Read the model definition and answer for the solid it produces. Units are mm, in the model's axes. Face numbers are marked on the shaded views. A direction names the side the tool comes from. Give positions to 0.01 mm unless a question says otherwise; leave off trailing zeros. Order: outer loops, then holes, each group sorted by start corner. A loop starts at its lowest first (then second) coordinate and runs counter-clockwise, first axis right, second up.
Item 1: The mould has two halves that part along Y. Classify the marked faces 1, 2 and 3: +Y half, -Y half, draft (parallel to the pull), parting line (faces both ways), or undercut.
Item 2: A cutting plane is placed at D-D (z = 56). Write down the section's boundary in (x, y).
Item 3: A cutting plane is placed at A-A (z = 180). Write down the section's boundary in (x, y).
Item 4: A cutting plane is placed at C-C (x = 50). Write down the section's boundary in (y, z), plus the area to 3 significant figures.
Item 5: A cutting plane is placed at B-B (x = 440). Write down the section's boundary in (y, z), plus the area to 3 significant figures.
Item 6: Which of the six approach directions +Z, -Z, +X, -X, +Y, -Y give full straight-line access (tool end or side, diameter ignored) to the marked faces 4, 5 and 6?
Item 7: Find the intervals of material crossed by line 1 along Y through (x, z) = (440, 170); line 2 along Z through (x, y) = (50, 96.25); line 3 along Z through (x, y) = (50, 30), in increasing order.
Item 8: Given pin 1 Ø8 at (y, z) = (165, 27) entering from +X; pin 2 Ø5 at (x, z) = (305, 47.5) entering from +Y; pin 3 Ø1 at (x, z) = (162, 186) entering from -Y, each flat-ended and moving along its own axis, determine where each tip first touches the part or whether it passes through.
Autodesk Inventor part; units mm, degrees
ref_plane "YZ Plane" through (0, 0, 0) normal (1, 0, 0) x (0, 1, 0)
ref_plane "XZ Plane" through (0, 0, 0) normal (0, 1, 0) x (-1, 0, 0)
ref_plane "XY Plane" through (0, 0, 0) normal (0, 0, 1) x (1, 0, 0)
sketch "Sketch1" plane through (0, 0, 0) normal (0, 0, 1) x (1, 0, 0)
  line L0 (0, 0) -> (0, 100)
  line L1 (0, 100) -> (200, 100)
  line L2 (500, 150) -> (500, 0)
  line L3 (500, 0) -> (300, 0)
  line L4 (300, 0) -> (300, -40)
  line L5 (300, -40) -> (200, -40)
  line L6 (200, -40) -> (200, 0)
  line L7 (200, 0) -> (0, 0)
  circle A0 centre (440, 75) radius 18.75
  arc A1 (191.2122, 100) -> (371.4743, 150) centre (250, 238) ccw
  line L8 (371.4743, 150) -> (500, 150)
  line L9 (362.8128, 194) -> (388.2162, 150)
  line L10 (255.4256, 132) -> (270.4256, 106.0192)
  line L11 (270.4256, 106.0192) -> (322.3872, 136.0192)
  line L12 (322.3872, 136.0192) -> (307.3872, 162)
  line L13 (200, 100) -> (255.4256, 132)
  line L14 (307.3872, 162) -> (362.8128, 194)
  dimension "d0" = 100
  dimension "d2" = 200
  dimension "d3" = 100
  dimension "d4" = 40
  dimension "d5" = 150
  dimension "d6" = 75
  dimension "d7" = 60
  dimension "d8" = 37.5
  dimension "d10" = 250
  dimension "d11" = 200
  dimension "d12" = 138
  dimension "d13" = 150
  dimension "d15" = 188
  dimension "d16" = 60
  dimension "d17" = 30
  dimension "d18" = 30
  dimension "d19" = 500
extrude "Extrusion1" add sketch "Sketch1" along normal blind 230 contours L0 L1 A1 L8 L2 L3 L4 L5 L6 L7
extrude "Extrusion2" add sketch "Sketch1" along normal blind 140 contours L1 L13 L10 L11 L12 L14 L9 L8 A1
sketch "Sketch2" plane through (0, 100, 230) normal (0, 1, 0) x (1, 0, 0)
  line L0 (0, 230) -> (0, 0)
  line L1 (50, 180) -> (50, 50) construction
  point P0 (50, 115)
  point P1 (0, 115)
  dimension "d24" = 50
  dimension "d25" = 130
hole "Hole1" at (50, 100, 50) at (50, 100, 180) direction (0, -1, 0) diameter 30 depth 100 counterbore diameter 50 counterbore depth 10
sketch "Sketch3" plane through (307.3872, 162, 140) normal (-0.5, 0.8660254, 0) x (0.8660254, 0.5, 0)
  line L0 (64, 140) -> (64, 0)
  line L1 (-60, 140) -> (-124, 140)
  line L2 (-124, 140) -> (-124, 0)
  line L3 (-60, 0) -> (-124, 0)
  line L4 (-60, 140) -> (-60, 0)
  line L5 (0, 140) -> (-60, 140)
  line L6 (-60, 140) -> (-60, 0)
  line L7 (0, 0) -> (-60, 0)
  line L8 (0, 140) -> (0, 0)
  circle A0 centre (-30, 70) radius 50
  line L9 (-30, 0) -> (-30, 140) construction
  line L10 (64, 70) -> (-124, 70) construction
  point P0 (-347.2051, 140)
  point P1 (-102, 110)
  point P2 (-102, 30)
  point P3 (42, 110)
  point P4 (42, 30)
  dimension "d33" = 100
  dimension "d34" = 80
hole "Hole2" at (219.0526, 111, 30) at (219.0526, 111, 110) at (343.7602, 183, 30) at (343.7602, 183, 110) direction (0.5, -0.8660254, 0) diameter 18.5 depth 20 tip angle 118
extrude "Extrusion3" cut sketch "Sketch3" against normal blind 15 contours A0 L8 L4 | L4 A0 | A0 L8
properties part number "b3"
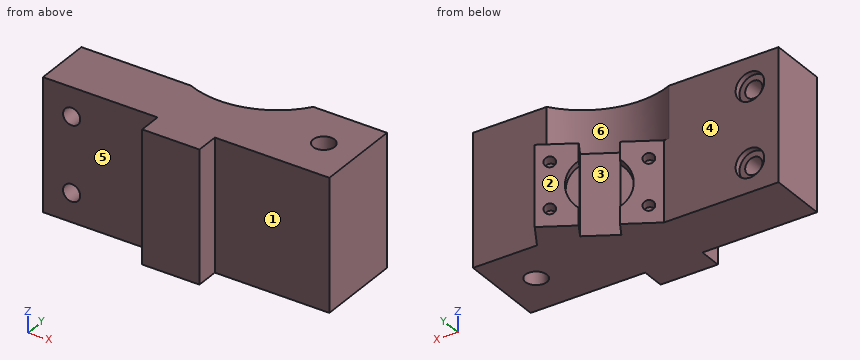
Response values:
1. face 1: -Y half
1. face 2: +Y half
1. face 3: undercut
2. outline: (0, 0) - (36.25, 0) - (36.25, 90) - (25.73, 90) - (25.73, 100) - (0, 100) - close; (63.75, 0) - (200, 0) - (200, -40) - (300, -40) - (300, 0) - (500, 0) - (500, 150) - (388.22, 150) - (362.81, 194) - (322.98, 171) - (330.48, 158.01) - (314.89, 149.01) - (322.39, 136.02) - (270.43, 106.02) - (262.93, 119.01) - (247.34, 110.01) - (239.84, 123) - (200, 100) - (74.27, 100) - (74.27, 90) - (63.75, 90) - close; hole circle Ø37.5 at (440, 75)
3. outline: (0, 0) - (35, 0) - (35, 90) - (25, 90) - (25, 100) - (0, 100) - close; (65, 0) - (200, 0) - (200, -40) - (300, -40) - (300, 0) - (500, 0) - (500, 150) - (371.47, 150) arc R150 cw to (191.21, 100) - (75, 100) - (75, 90) - (65, 90) - close; hole circle Ø37.5 at (440, 75)
4. outline: (0, 0) - (100, 0) - (100, 25) - (90, 25) - (90, 35) - (0, 35) - close; (0, 65) - (90, 65) - (90, 75) - (100, 75) - (100, 155) - (90, 155) - (90, 165) - (0, 165) - close; (0, 195) - (90, 195) - (90, 205) - (100, 205) - (100, 230) - (0, 230) - close
4. area: 16,600 mm2
5. outline: (0, 0) - (56.25, 0) - (56.25, 230) - (0, 230) - close; (93.75, 0) - (150, 0) - (150, 230) - (93.75, 230) - close
5. area: 25,900 mm2
6. face 4: +Z, -Z, -X, +Y
6. face 5: +Z, -Z, -X, -Y
6. face 6: +Z, +Y
7. line 1: y = 0 to 56.25, 93.75 to 150
7. line 2: z = 0 to 25, 75 to 155, 205 to 230
7. line 3: z = 0 to 35, 65 to 165, 195 to 230
8. pin 1: stops at x = 381.87
8. pin 2: stops at y = 127.42
8. pin 3: stops at y = 0
